```python
from build123d import *

# Parameters (mm, degrees)
SKETCH003_R             = 5.588
PAD003_DEPTH            = 9.0932
SKETCH004_W             = 1.9431
SKETCH004_H             = 3.2639
PAD004_DEPTH            = 0.508
BODY003_PLACEMENT_ANGLE = 90
SKETCH005_W             = 25.4
SKETCH005_H             = 38.1
SKETCH005_R             = 1.9304
SKETCH005_R_2           = 0.9906
PAD005_DEPTH            = 1.5875
SKETCH_W                = 5.9944
SKETCH_H                = 14.478
PAD_DEPTH               = 5.08
SKETCH001_R             = 2.5019
SKETCH001_R_2           = 1.7399
PAD001_DEPTH            = 2.4892
SKETCH002_R             = 0.7493
PAD002_DEPTH            = 1.016


with BuildPart() as switch_clone:
    # Sketch003 → Pad003 (new body)
    with BuildSketch(Plane.XY):
        Circle(SKETCH003_R)
    extrude(amount=PAD003_DEPTH)

    # Sketch004 (on Face2 of Pad003) → Pad004 (join)
    with BuildSketch(Plane(origin=(0, 0, 0), x_dir=(1, 0, 0), z_dir=(0, 0, -1))):
        with Locations((-2.36855, 4.17195)):
            Rectangle(SKETCH004_W, SKETCH004_H)
        with Locations((2.36855, 4.17195)):
            Rectangle(SKETCH004_W, SKETCH004_H)
        with Locations((2.36855, -4.17195)):
            Rectangle(SKETCH004_W, SKETCH004_H)
        with Locations((-2.36855, -4.17195)):
            Rectangle(SKETCH004_W, SKETCH004_H)
    extrude(amount=-PAD004_DEPTH)


with BuildPart() as switch_clone_1:
    # Body003 placement: moved
    add(switch_clone.part.moved(Location((0, 25.4, 0))).rotate(Axis((0, 25.4, 0), (0, 0, 1)), BODY003_PLACEMENT_ANGLE))


with BuildPart() as bare_pcb_clone:
    # Sketch005 → Pad005 (new body)
    with BuildSketch(Plane.XY):
        with Locations((0, 19.05)):
            Rectangle(SKETCH005_W, SKETCH005_H)
        with Locations((-8.89, 3.81)):
            Circle(SKETCH005_R, mode=Mode.SUBTRACT)
        with Locations((8.89, 34.29)):
            Circle(SKETCH005_R, mode=Mode.SUBTRACT)
        with Locations((0, 3.175)):
            Circle(SKETCH005_R_2, mode=Mode.SUBTRACT)
        with Locations((0, 10.16)):
            Circle(SKETCH005_R_2, mode=Mode.SUBTRACT)
    extrude(amount=-PAD005_DEPTH)


with BuildPart() as populated_pcb_clone:
    # Sketch → Pad (new body)
    with BuildSketch(Plane.XY):
        with Locations((0, 7.239)):
            Rectangle(SKETCH_W, SKETCH_H)
    extrude(amount=PAD_DEPTH)

    # Sketch001 (on Face3 of Pad) → Pad001 (join)
    with BuildSketch(Plane.XZ):
        with Locations((0, 2.54)):
            Circle(SKETCH001_R)
        with Locations((0, 2.54)):
            Circle(SKETCH001_R_2, mode=Mode.SUBTRACT)
    extrude(amount=PAD001_DEPTH)

    # Sketch002 (on Face4 of Pad001) → Pad002 (join)
    with BuildSketch(Plane(origin=(0, 0, 0), x_dir=(1, 0, 0), z_dir=(0, 0, -1))):
        with Locations((0, -3.5052)):
            Circle(SKETCH002_R)
        with Locations((0, -10.5156)):
            Circle(SKETCH002_R)
    extrude(amount=PAD002_DEPTH)


with BuildPart() as populated_pcb_clone_1:
    # Body002 placement: moved
    add(populated_pcb_clone.part.moved(Location((0, -0.3302, 0))))

    # Fusion: union switch clone, bare pcb clone
    add(switch_clone_1.part)
    add(bare_pcb_clone.part)


with BuildPart() as populated_pcb_clone_2:
    # Body006 placement: moved
    add(populated_pcb_clone_1.part.moved(Location((0, 0, -2.54))))


solid = populated_pcb_clone_2.part
```
CAD build for the part. Positions are in the model's coordinates, mm. A direction names the side the tool comes from. Coordinates: 2 decimals unless noted, no trailing zeros. Order: outer loops, then holes, each group sorted by start corner. A loop starts at its lowest first (then second) coordinate and runs counter-clockwise, first axis right, second up. Notation, with made-up numbers: (75.25, 2) - (86.25, 2) arc R29 cw to (86.25, 27) - close; hole circle Ø9 at (-22.75, -35.75). An arc over 180 degrees is marked (long way). Use a Markdown table: item, result. Add a question column.
(1) Saw through at C-C (y = 25.4). Give the cut face in (x, z).
(2) Saw through at D-D (x = -5). Give the cut face in (y, z).
(3) Flat gauge pins, fed straight in: pin 1 (3 mm diameter, centred on x = -8.89, y = 3.81, fed in from +Z); pin 2 (3 mm diameter, centred on x = 0.5, z = 0, fed in from +Y); pin 3 (3 mm diameter, centred on y = 12, z = 0, fed in from -X); pin 4 (5 mm diameter, centred on x = -4, z = 4, fed in from +Y). Where does each tip first touch, or does it go through?
(4) Which spindle directions (+Z, -Z, +X, -X, +Y, -Y) get a long thin tool onto all of the face, cutting with end or side? Do faces 1 (the face through (-5.4, 28, -2.032)), 2 (the face through (5.3, 22.8, -2.032)), 3 (the face through (-0.542, -1.557, -2.442)), 4 (the face through (-2.997, 7, 0)), 5 (the face through (0, 3, -3.556)). Say none if no direction does.
(5) Saw through at A-A (y = 34.29). Give the cut face in (x, z).
(6) Drill centre lines: line 1 along Y through (x, z) = (0, -3.4); line 2 along Y through (x, z) = (8.89, -3.2); line 3 along Z through (x, y) = (4.75, 8.5). Where is each one in solid material? Low to high. Write a range as [from, to].
(7) Pull direction Y, two halves, no side cores. Call faces 6 (the face through (0, 10, -3.556)), 7 (the face through (-1.38, -1.56, -1.06)), 8 (the face through (0, 38.1, -3)): +Y half, -Y half, draft (parallel to the pull), parting line (faces both ways), or undercut.
(8) Saw through at B-B (x = -8.89). Give the cut face in (y, z).
Solved:
| question | item | result |
|---|---|---|
| 1 | outline | (-12.7, -4.13) - (12.7, -4.13) - (12.7, -2.54) - (5.59, -2.54) - (5.59, 6.55) - (-5.59, 6.55) - (-5.59, -2.54) - (-12.7, -2.54) - close |
| 2 | outline | (0, -4.13) - (38.1, -4.13) - (38.1, -2.54) - (28.74, -2.54) - (28.74, -2.03) - (27.9, -2.03) - (27.9, 6.55) - (22.9, 6.55) - (22.9, -2.03) - (22.06, -2.03) - (22.06, -2.54) - (0, -2.54) - close |
| 3 | pin 1 | passes through |
| 3 | pin 2 | stops at y = 30.99 |
| 3 | pin 3 | stops at x = -3 |
| 3 | pin 4 | stops at y = 30.78 |
| 4 | face 1 | +Z, -X, +Y |
| 4 | face 2 | +Z, +X, -Y |
| 4 | face 3 | -Y |
| 4 | face 4 | +Z, -X, -Y |
| 4 | face 5 | -Z |
| 5 | outline | (-12.7, -4.13) - (6.96, -4.13) - (6.96, -2.54) - (-12.7, -2.54) - close; (10.82, -4.13) - (12.7, -4.13) - (12.7, -2.54) - (10.82, -2.54) - close |
| 6 | line 1 | y = [0, 2.18], [2.43, 3.92], [4.17, 9.17], [9.44, 10.93], [11.15, 38.1] |
| 6 | line 2 | y = [0, 32.36], [36.22, 38.1] |
| 6 | line 3 | z = [-4.13, -2.54] |
| 7 | face 6 | undercut |
| 7 | face 7 | draft |
| 7 | face 8 | +Y half |
| 8 | outline | (0, -4.13) - (1.88, -4.13) - (1.88, -2.54) - (0, -2.54) - close; (5.74, -4.13) - (38.1, -4.13) - (38.1, -2.54) - (5.74, -2.54) - close |
